```python
from build123d import *

# Parameters (mm, degrees)
F0_W        = 80
F0_H        = 6.5
F1_DEPTH    = 2
F0_H_2      = 2
F2_DEPTH    = 13
F3_W        = 1.5
F3_H        = 3
F4_DEPTH    = 80
F5_R        = 1
F6_R        = 1
F7_T1_DEPTH = 80
F8_R        = 0.5
F9_DEPTH    = 0.5


# Not quite as in the source:
# - a fillet or chamfer that OpenCascade refuses, or shapes differently, is made with other operations: its cross-section is extruded or revolved along the edge and cut away or added
# - a feature names something its author has since deleted; it is built from what else it names


with BuildPart() as f1:
    # F0 (on Top) → F1 (new body)
    with BuildSketch(Plane.XY):
        Rectangle(F0_W, F0_H)
    extrude(amount=F1_DEPTH)

    # F0 (on Top) → F2 (join)
    with BuildSketch(Plane.XY):
        with Locations((0, 4.25)):
            Rectangle(F0_W, F0_H_2)
        with Locations((0, -4.25)):
            Rectangle(F0_W, F0_H_2)
    extrude(amount=F2_DEPTH)

    # F3 (on face) → F4 (join)
    with BuildSketch(Plane(origin=(-40, 0, 0), x_dir=(0, -1, 0), z_dir=(-1, 0, 0))):
        Polygon((-3.25, 13), (-3.25, 9), (-2.55, 11), align=None)
        Polygon((2.55, 11), (3.25, 9), (3.25, 13), align=None)
        with Locations((0, 3.5)):
            Rectangle(F3_W, F3_H)
    extrude(amount=-F4_DEPTH)

    # F5
    f5_edges = [f1.edges().sort_by_distance(p)[0] for p in [
        (0, 2.55, 11),
    ]]
    fillet(f5_edges, radius=F5_R)

    # F6
    f6_edges = [f1.edges().sort_by_distance(p)[0] for p in [
        (0, -2.55, 11),
    ]]
    fillet(f6_edges, radius=F6_R)

    # F7: fillet of radius 1.5 on 4 edges, made by hand

    # F7_s2 → F7_t1 (join)
    with BuildSketch(Plane.YZ.offset(-40)):
        with BuildLine():
            ThreePointArc((-3.25, 3.5), (-2.8106601718, 2.4393398282), (-1.75, 2))
            Line((-1.75, 2), (-3.25, 2))
            Line((-3.25, 2), (-3.25, 3.5))
        make_face()
        with BuildLine():
            ThreePointArc((1.75, 2), (2.8106601718, 2.4393398282), (3.25, 3.5))
            Line((3.25, 3.5), (3.25, 2))
            Line((3.25, 2), (1.75, 2))
        make_face()
        with BuildLine():
            ThreePointArc((-2.25, 2), (-1.1893398282, 2.4393398282), (-0.75, 3.5))
            Line((-0.75, 3.5), (-0.75, 2))
            Line((-0.75, 2), (-2.25, 2))
        make_face()
        with BuildLine():
            ThreePointArc((0.75, 3.5), (1.1893398282, 2.4393398282), (2.25, 2))
            Line((2.25, 2), (0.75, 2))
            Line((0.75, 2), (0.75, 3.5))
        make_face()
    extrude(amount=F7_T1_DEPTH)

    # F8
    f8_edges = [f1.edges().sort_by_distance(p)[0] for p in [
        (0, -0.75, 5),
        (0, 0.75, 5),
        (-40, 0, 5),
        (40, 0, 5),
    ]]
    fillet(f8_edges, radius=F8_R)

    # F0 (on Top) → F9 (join)
    with BuildSketch(Plane.XY):
        with BuildLine():
            ThreePointArc((50.4157468677, 5.4975104332), (48.9512807736, 9.0330443391), (45.4157468677, 10.4975104332))
            Line((45.4157468677, 10.4975104332), (-45.4157468677, 10.4975104332))
            ThreePointArc((-45.4157468677, 10.4975104332), (-48.9512807736, 9.0330443391), (-50.4157468677, 5.4975104332))
            Line((-50.4157468677, 5.4975104332), (-50.4157468677, -5.4975104332))
            ThreePointArc((-50.4157468677, -5.4975104332), (-48.9512807736, -9.0330443391), (-45.4157468677, -10.4975104332))
            Line((-45.4157468677, -10.4975104332), (45.4157468677, -10.4975104332))
            ThreePointArc((45.4157468677, -10.4975104332), (48.9512807736, -9.0330443391), (50.4157468677, -5.4975104332))
            Line((50.4157468677, -5.4975104332), (50.4157468677, 5.4975104332))
        make_face()
        Polygon((-40, 5.25), (40, 5.25), (40, 3.25), (40, -3.25), (40, -5.25), (-40, -5.25), (-40, -3.25), (-40, 3.25), align=None, mode=Mode.SUBTRACT)
    extrude(amount=F9_DEPTH)


solid = f1.part
```
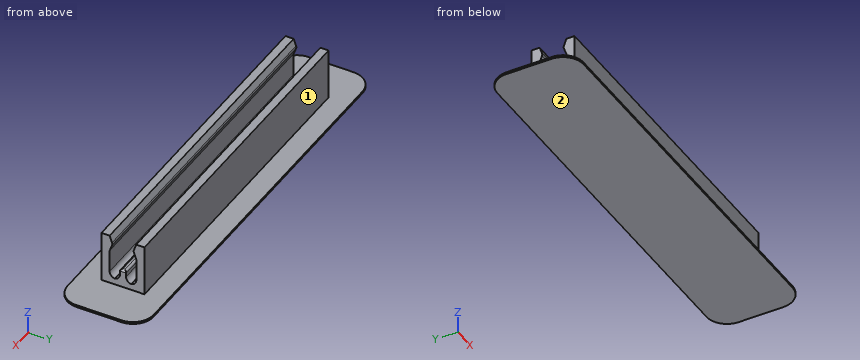
Verification items for the finished model (mm, model axes). Face numbers are marked on the shaded views. A direction names the side the tool comes from. Round coordinates to 2 decimals unless told otherwise and drop trailing zeros. Order: outer loops, then holes, each group sorted by start corner. A loop starts at its lowest first (then second) coordinate and runs counter-clockwise, first axis right, second up. Notation, with made-up numbers: (-18, 73) -> (4, 73) arc R33 cw to (4, 107) -> close; hole circle Ø9 at (-32.75, -38.5). An arc over 180 degrees is marked (long way). Put each result on its own line as item: value. Start each with the question number.
(1) Section check D-D (x = 43). Enter the section's corners in (y, z), then the cut area to 3 significant figures.
(2) Material ranges on line 1 along Y through (x, z) = (-23, 3.75); line 2 along Y through (x, z) = (23, 5.5); line 3 along X through (y, z) = (5, 9), recorded low to high.
(3) Section check A-A (z = 6.75). Enter the section's corners in (x, y), then the cut area to 3 significant figures.
(4) Depth check by flat-ended pin: pin 1 Ø6 at (x, z) = (2.5, 2.5) entering from -Y; pin 2 Ø1.1 at (x, z) = (19, 4) entering from +Y; pin 3 Ø5 at (y, z) = (-1, 8.5) entering from -X; pin 4 Ø4.5 at (x, z) = (7, 7) entering from -Y. Enter the tip coordinate at first touch or a pass-through.
(5) Tool access check on the marked faces 1 and 2. Record the directions out of +Z, -Z, +X, -X, +Y, -Y that give a thin tool (end or side, any length) a straight path to the whole face; none if there is none.
(6) Section check C-C (y = 7.5). Enter the section's corners in (x, z).
(7) Section check B-B (x = 22). Enter the section's corners in (y, z).
Completed:
1. outline: (-10.5, 0) -> (10.5, 0) -> (10.5, 0.5) -> (-10.5, 0.5) -> close
1. area: 10.5 mm2
2. line 1: y = -5.25 to -3.25, -0.75 to 0.75, 3.25 to 5.25
2. line 2: y = -5.25 to -3.25, 3.25 to 5.25
2. line 3: x = -40 to 40
3. outline: (-40, -5.25) -> (40, -5.25) -> (40, -3.25) -> (-40, -3.25) -> close; (-40, 3.25) -> (40, 3.25) -> (40, 5.25) -> (-40, 5.25) -> close
3. area: 320 mm2
4. pin 1: stops at y = -10.5
4. pin 2: stops at y = 5.25
4. pin 3: stops at x = -40
4. pin 4: stops at y = -5.25
5. face 1: +Z, +X, -X, +Y
5. face 2: -Z, +X, -X, +Y, -Y
6. outline: (-50, 0) -> (50, 0) -> (50, 0.5) -> (-50, 0.5) -> close
7. outline: (-10.5, 0) -> (10.5, 0) -> (10.5, 0.5) -> (5.25, 0.5) -> (5.25, 13) -> (3.25, 13) -> (2.67, 11.33) arc R1 ccw to (2.67, 10.67) -> (3.25, 9) -> (3.25, 3.5) arc R1.5 cw to (2, 2.02) arc R1.5 cw to (0.75, 3.5) -> (0.75, 4.5) arc R0.5 ccw to (0.25, 5) -> (-0.25, 5) arc R0.5 ccw to (-0.75, 4.5) -> (-0.75, 3.5) arc R1.5 cw to (-2, 2.02) arc R1.5 cw to (-3.25, 3.5) -> (-3.25, 9) -> (-2.67, 10.67) arc R1 ccw to (-2.67, 11.33) -> (-3.25, 13) -> (-5.25, 13) -> (-5.25, 0.5) -> (-10.5, 0.5) -> close
